Answer from the drawing. Dimensions are ordinates in mm from the lowest x, y and z of the part. A direction names the side the tool comes from. Coordinates: 2 decimals unless noted, no trailing zeros. Order: outer loops, then holes, each group sorted by start corner. A loop starts at its lowest first (then second) coordinate and runs counter-clockwise, first axis right, second up. Notation, with made-up numbers: (-32.75, 21) -> (-26.75, 21) arc R25 ccw to (-26.75, 37) -> close; hole circle Ø9 at (31.25, 52). An arc over 180 degrees is marked (long way). Answer in a Markdown table with one row per item.
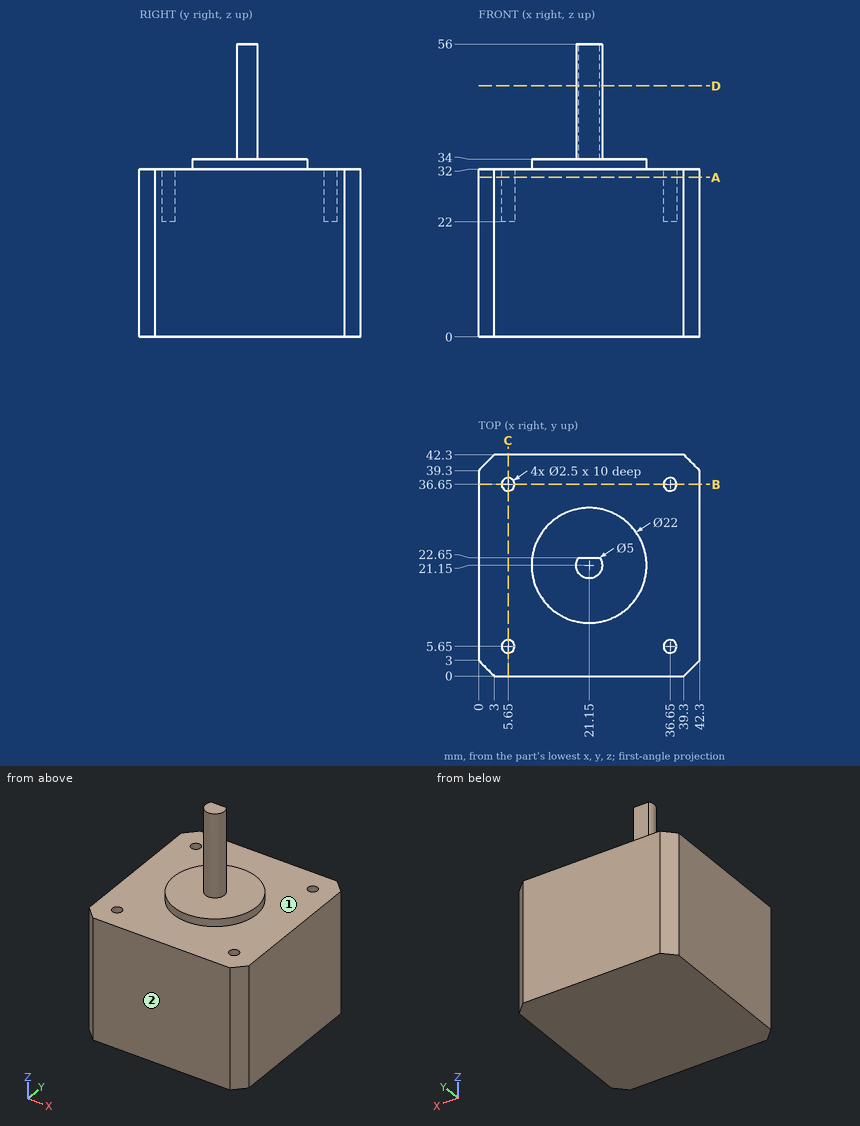
(1) A cutting plane is placed at D-D, the plane z = 48. Determine the outline of the cut face in (x, y).
Check values:
| item | result |
|---|---|
| outline | (19.15, 22.65) arc R2.5 ccw (long way) to (23.15, 22.65) -> close |
(2) A cutting plane is placed at A-A, the plane z = 30.5. Determine the outline of the cut face in (x, y).
Check values:
| item | result |
|---|---|
| outline | (0, 3) -> (3, 0) -> (39.3, 0) -> (42.3, 3) -> (42.3, 39.3) -> (39.3, 42.3) -> (3, 42.3) -> (0, 39.3) -> close; hole circle Ø2.5 at (5.65, 5.65); hole circle Ø2.5 at (5.65, 36.65); hole circle Ø2.5 at (36.65, 5.65); hole circle Ø2.5 at (36.65, 36.65) |
(3) Find the intervals of material crossed by line 1 along X through (y, z) = (36, 25); line 2 along Z through (x, y) = (24.5, 31.5); line 3 along Z through (x, y) = (3, 31), in increasing order. Write a range as from..to.
Check values:
| item | result |
|---|---|
| line 1 | 0..4.58, 6.72..35.58, 37.72..42.3 |
| line 2 | 0..34 |
| line 3 | 0..32 |
(4) A cutting plane is placed at B-B, the plane y = 36.65. Determine the outline of the cut face in (x, z), then the cut area to 3 significant figures.
Check values:
| item | result |
|---|---|
| outline | (0, 0) -> (42.3, 0) -> (42.3, 32) -> (37.9, 32) -> (37.9, 22) -> (35.4, 22) -> (35.4, 32) -> (6.9, 32) -> (6.9, 22) -> (4.4, 22) -> (4.4, 32) -> (0, 32) -> close |
| area | 1,300 mm² |
(5) Which of the six approach directions +Z, -Z, +X, -X, +Y, -Y give full straight-line access (tool end or side, diameter ignored) to the marked faces 1 and 2?
Check values:
| item | result |
|---|---|
| face 1 | +Z |
| face 2 | +Z, -Z, +X, -X, -Y |
(6) Flat-ended cylindrical pins translate along their axes: pin 1 (3 mm diameter, centred on x = 21, z = 50, fed in from +Y); pin 2 (3 mm diameter, centred on x = 37, y = 6, fed in from +Z); pin 3 (6 mm diameter, centred on y = 8.5, z = 16.5, fed in from -X); pin 4 (2 mm diameter, centred on x = 5.65, y = 36.65, fed in from +Z). Find the tip coordinate at first contact, or state that the pin passes through.
Check values:
| item | result |
|---|---|
| pin 1 | y = 22.65 |
| pin 2 | z = 32 |
| pin 3 | x = 0 |
| pin 4 | z = 22 |
